For this review, take the finished solid that the model builds, in its own axes (mm). Give positions to 0.01 mm unless a question says otherwise; leave off trailing zeros. Order: outer loops, then holes, each group sorted by start corner. A loop starts at its lowest first (then second) coordinate and runs counter-clockwise, first axis right, second up. Notation, with made-up numbers: (37.25, 49.5) - (48.25, 49.5) arc R16 cw to (48.25, 78.5) - close; hole circle Ø3 at (79.25, 21). An arc over 180 degrees is marked (long way). Put each result on its own line as item: value. Start each with the question number.
```python
from build123d import *

# Parameters (mm, degrees)
SKETCH1_R           = 30
SKETCH1_R_2         = 1.5
SKETCH1_W           = 3
SKETCH1_H           = 5
BOSS_EXTRUDE1_DEPTH = 1


with BuildPart() as part:
    # Sketch1 → Boss-Extrude1 (new body)
    with BuildSketch(Plane.XY):
        with BuildLine():
            Line((-73.593555797, 14.456436117), (-18, -72.807966597))
            ThreePointArc((-18, -72.807966597), (0, -75), (18, -72.807966597))
            Line((18, -72.807966597), (73.593555797, 14.456436117))
            ThreePointArc((73.593555797, 14.456436117), (67.973084028, 31.696369631), (58.379298374, 47.083516451))
            Line((58.379298374, 47.083516451), (-58.379298374, 47.083516451))
            ThreePointArc((-58.379298374, 47.083516451), (-67.973084028, 31.696369631), (-73.593555797, 14.456436117))
        make_face()
        Circle(SKETCH1_R, mode=Mode.SUBTRACT)
        with Locations((0, -43)):
            Circle(SKETCH1_R_2, mode=Mode.SUBTRACT)
        with Locations((-37.239092363, -21.5)):
            Circle(SKETCH1_R_2, mode=Mode.SUBTRACT)
        with Locations((-37.239092363, 21.5)):
            Circle(SKETCH1_R_2, mode=Mode.SUBTRACT)
        with Locations((0, 43)):
            Circle(SKETCH1_R_2, mode=Mode.SUBTRACT)
        with Locations((37.239092363, 21.5)):
            Circle(SKETCH1_R_2, mode=Mode.SUBTRACT)
        with Locations((37.239092363, -21.5)):
            Circle(SKETCH1_R_2, mode=Mode.SUBTRACT)
        with Locations((0, -60)):
            Circle(SKETCH1_R_2, mode=Mode.SUBTRACT)
        with Locations((54.378467222, 25.357095704)):
            Circle(SKETCH1_R_2, mode=Mode.SUBTRACT)
        with Locations((-54.378467222, 25.357095704)):
            Circle(SKETCH1_R_2, mode=Mode.SUBTRACT)
        with Locations((0, -52.5)):
            Rectangle(SKETCH1_W, SKETCH1_H, mode=Mode.SUBTRACT)
        with Locations((0, -67.5)):
            Rectangle(SKETCH1_W, SKETCH1_H, mode=Mode.SUBTRACT)
        Polygon((49.213000894, 24.603466076), (44.681461959, 22.490374768), (45.949316744, 19.771451406), (50.48085568, 21.884542715), align=None, mode=Mode.SUBTRACT)
        Polygon((58.276078765, 28.829648694), (62.8076177, 30.942740002), (64.075472485, 28.223816641), (59.54393355, 26.110725333), align=None, mode=Mode.SUBTRACT)
        Polygon((-58.276078765, 28.829648694), (-62.8076177, 30.942740002), (-64.075472485, 28.223816641), (-59.54393355, 26.110725333), align=None, mode=Mode.SUBTRACT)
        Polygon((-49.213000894, 24.603466076), (-44.681461959, 22.490374768), (-45.949316744, 19.771451406), (-50.48085568, 21.884542715), align=None, mode=Mode.SUBTRACT)
    extrude(amount=BOSS_EXTRUDE1_DEPTH)


solid = part.part
```
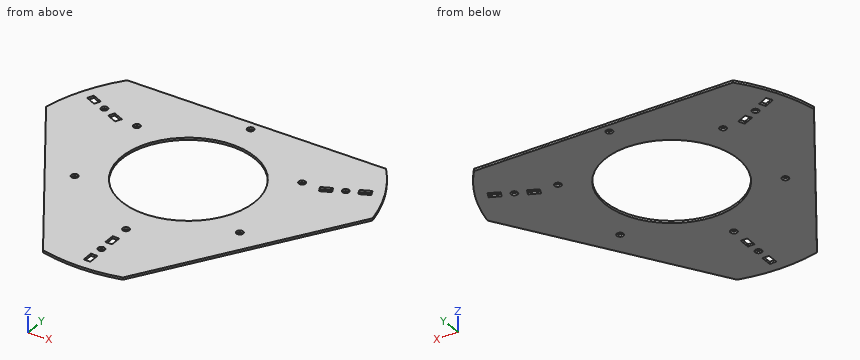
1. Add section A-A, the plane y = -9. Give the boundary of the cut face in (x, z), then the cut area to 3 significant figures.
2. Add section B-B, the plane z = 0.2. Count the separate pieces of the cut face and the enclosed holes in it, then the cut area to 3 significant figures.
3. Wall thickness on line 1 (X direction, y = 26.5, z = 0.55); line 2 (X direction, y = 22, z = 0.2); line 3 (Y direction, x = 10, z = 0.35): over which ranges is each line inside the solid? List them lowest first. Write a range as from..to.
4. Clearance check with flat-ended pins moving along their axes: pin 1 (12 mm diameter, centred on x = 47.5, y = -20.5, fed in from -Z); pin 2 (0.5 mm diameter, centred on x = 0, z = 0.5, fed in from -Y); pin 3 (0.5 mm diameter, centred on y = -67.5, z = 0.5, fed in from -X). State where each tip first meets the part, or that it passes through.
Found:
1. outline: (-58.65, 0) - (-28.62, 0) - (-28.62, 1) - (-58.65, 1) - close; (28.62, 0) - (58.65, 0) - (58.65, 1) - (28.62, 1) - close
1. area: 60.1 mm^2
2. separate pieces: 1
2. enclosed holes: 16
2. area: 9,480 mm^2
3. line 1: x = -70.16..-60.38, -59.36..-55.35, -53.41..-14.06, 14.06..53.41, 55.35..59.36, 60.38..70.16
3. line 2: x = -71.7..-50.43, -44.91..-38.65, -35.82..-20.4, 20.4..35.82, 38.65..44.91, 50.43..71.7
3. line 3: y = -74.33..-28.28, 28.28..47.08
4. pin 1: stops at z = 0
4. pin 2: stops at y = -75
4. pin 3: stops at x = -21.54
